```python
from build123d import *

# Parameters (mm, degrees)
F0_R     = 29.6395356571
F1_DEPTH = 7.62
F2_R     = 3.81
F3_R     = 3.80999


# Not quite as in the source:
# - a fillet or chamfer is up to 0.001 mm smaller than in the source, because OpenCascade refuses the exact size


with BuildPart() as f1:
    # F0 (on Top) → F1 (new body)
    with BuildSketch(Plane.XY):
        Circle(F0_R)
    extrude(amount=F1_DEPTH)

    # F2
    f2_edges = [f1.edges().sort_by_distance(p)[0] for p in [
        (-29.639536, 0, 7.62),
    ]]
    fillet(f2_edges, radius=F2_R)

    # F3 (radius 3.81 in the source; OpenCascade refuses exactly that, so slightly less here)
    f3_edges = [f1.edges().sort_by_distance(p)[0] for p in [
        (-29.639536, 0, 0),
    ]]
    fillet(f3_edges, radius=F3_R)


solid = f1.part
```
Input: part model. Units: mm. Frame: model coordinates. Coordinates: 2 decimals unless noted, no trailing zeros. Loops run counter-clockwise (first coordinate to the right, second up) from the corner with the lowest first, then second, coordinate; pieces in that order, holes last. Notation, with made-up numbers: M -32.5,11.5 L -1.5,11.5 A10 ccw -1.5,29.5 Z; hole C 3,4.25 d7. An arc over 180 degrees is marked long. Answer in a Markdown table with one row per item.
1. Section D-D, the plane z = 6.5. Output: boundary loops of the cut face in (x, y), then the cut area to 3 significant figures.
Response:
| item | result |
|---|---|
| outline | C 0,0 d57.06 |
| area | 2,560 mm2 |
2. Material intervals for line 1 (Y direction, x = -14.5, z = 3.75); line 2 (X direction, y = 20, z = 4.75); line 3 (X direction, y = 2, z = 1), sorted ascending.
Response:
| item | result |
|---|---|
| line 1 | y = -25.85 to 25.85 |
| line 2 | x = -21.71 to 21.71 |
| line 3 | x = -28.33 to 28.33 |
3. Section C-C, the plane z = 2.25. Output: boundary loops of the cut face in (x, y), then the cut area to 3 significant figures.
Response:
| item | result |
|---|---|
| outline | C 0,0 d58.61 |
| area | 2,700 mm2 |
4. First-contact query: pin 1 (1.5 mm diameter, centred on y = -23, z = 5.5, fed in from -X); pin 2 (4 mm diameter, centred on x = 1, z = 3.5, fed in from -Y). Flat tips, straight axial feed; report the tip coordinate or a pass-through.
Response:
| item | result |
|---|---|
| pin 1 | stops at x = -19.11 |
| pin 2 | stops at y = -29.64 |
